```python
from build123d import *

# Parameters (mm, degrees)
EXTRUDE_THIN1_DEPTH  = 17
BOSS_EXTRUDE1_DEPTH  = 17
BOSS_EXTRUDE3_START  = 18
BOSS_EXTRUDE3_DEPTH  = 18
BOSS_EXTRUDE10_START = 18
BOSS_EXTRUDE10_DEPTH = 18
SKETCH6_W            = 4
SKETCH6_H            = 8
CUT_EXTRUDE1_DEPTH   = 1
BOSS_EXTRUDE4_DEPTH  = 18
CUT_EXTRUDE3_START   = -18
CUT_EXTRUDE3_DEPTH   = 18
BOSS_EXTRUDE5_DEPTH  = 17
BOSS_EXTRUDE6_DEPTH  = 2
SKETCH12_W           = 5
SKETCH12_H           = 1
BOSS_EXTRUDE8_DEPTH  = 33
SKETCH15_W           = 11.8
SKETCH15_H           = 8
CUT_EXTRUDE4_DEPTH   = 1
FILLET1_R            = 2
SKETCH16_W           = 30
SKETCH16_H           = 2
BOSS_EXTRUDE11_DEPTH = 18
BOSS_EXTRUDE12_START = -35
BOSS_EXTRUDE12_DEPTH = 35
SKETCH18_W           = 30
SKETCH18_H           = 35
CUT_EXTRUDE5_DEPTH   = 0.5
BOSS_EXTRUDE13_DEPTH = 2.7
BOSS_EXTRUDE14_START = -19.7
BOSS_EXTRUDE14_DEPTH = 19.7
SKETCH22_W           = 1
SKETCH22_H           = 18
BOSS_EXTRUDE15_DEPTH = 2
BOSS_EXTRUDE16_DEPTH = 19.7
BOSS_EXTRUDE17_DEPTH = 18
FILLET2_R            = 1
FILLET3_R            = 1
FILLET4_R            = 2
FILLET5_R            = 2
FILLET6_R            = 2


# Read off the part's stored shape, not the designer's step: Extrude-Thin1
with BuildPart() as part:
    # Extrude-Thin1 outline → Extrude-Thin1 (new body)
    with BuildSketch(Plane(origin=(0, 0, 0), x_dir=(1, 0, 0), z_dir=(0, 1, 0))):
        with BuildLine():
            Line((-13.736803788, -12.452377644), (-7.480049307, -32.917299422))
            Line((-7.480049307, -32.917299422), (-5.567439795, -32.332556012))
            Line((-5.567439795, -32.332556012), (-11.824194276, -11.867634235))
            ThreePointArc((-11.824194276, -11.867634235), (-11.857842102, -11.27507721), (-11.614075704, -10.733935872))
            Line((-11.614075704, -10.733935872), (-2, 1.571519877))
            Line((-2, 1.571519877), (-2, -2))
            Line((-2, -2), (32, -2))
            Line((32, -2), (32, 2.05634332))
            Line((32, 2.05634332), (34.813889941, 0.919457988))
            Line((34.813889941, 0.919457988), (35.563103127, 2.773825697))
            Line((35.563103127, 2.773825697), (30, 5.021465257))
            Line((30, 5.021465257), (30, 0))
            Line((30, 0), (0, 0))
            Line((0, 0), (0, 6.1))
            Line((0, 6.1), (-1, 6.1))
            Line((-1, 6.1), (-13.190097211, -9.502612921))
            ThreePointArc((-13.190097211, -9.502612921), (-13.824351917, -10.910606158), (-13.736803788, -12.452377644))
        make_face()
    extrude(amount=EXTRUDE_THIN1_DEPTH)

    # Sketch2 → Boss-Extrude1 (add)
    with BuildSketch(Plane(origin=(0, 17, 0), x_dir=(1, 0, 0), z_dir=(0, 1, 0))):
        Polygon((32, -2), (32, 2.05634332), (34.813889941, 0.919457988), align=None)
        Polygon((-2, -2), (-2, 1.571519877), (-5.158478254, -2.471147935), align=None)
    extrude(amount=-BOSS_EXTRUDE1_DEPTH)

    # Sketch5 → Boss-Extrude3 (add)
    with BuildSketch(Plane.XZ.offset(BOSS_EXTRUDE3_START)):
        with BuildLine():
            Line((-2, 2), (-5.158478254, 2.471147935))
            Line((-5.158478254, 2.471147935), (-11.614075704, 10.733935872))
            ThreePointArc((-11.614075704, 10.733935872), (-11.857842102, 11.27507721), (-11.824194276, 11.867634235))
            Line((-11.824194276, 11.867634235), (-5.567439795, 32.332556012))
            Line((-5.567439795, 32.332556012), (-6.523744551, 32.624927717))
            Line((-6.523744551, 32.624927717), (-12.780499032, 12.160005939))
            ThreePointArc((-12.780499032, 12.160005939), (-12.84109701, 11.092841684), (-12.402086458, 10.118274397))
            Line((-12.402086458, 10.118274397), (0, -5.755672387))
            Line((0, -5.755672387), (0, 2))
            Line((0, 2), (-2, 2))
        make_face()
    extrude(amount=-BOSS_EXTRUDE3_DEPTH)

    # Sketch14 → Boss-Extrude10 (add)
    with BuildSketch(Plane.XZ.offset(BOSS_EXTRUDE10_START)):
        with BuildLine():
            Line((0, -6.1), (-1, -6.1))
            Line((-1, -6.1), (-13.190097211, 9.502612921))
            ThreePointArc((-13.190097211, 9.502612921), (-13.824351917, 10.910606159), (-13.736803788, 12.452377644))
            Line((-13.736803788, 12.452377644), (-12.780499032, 12.160005939))
            ThreePointArc((-12.780499032, 12.160005939), (-12.84109701, 11.092841684), (-12.402086458, 10.118274397))
            Line((-12.402086458, 10.118274397), (0, -5.755672387))
            Line((0, -5.755672387), (0, -6.1))
        make_face()
    extrude(amount=-BOSS_EXTRUDE10_DEPTH)

    # Sketch6 → Cut-Extrude1 (cut)
    with BuildSketch(Plane(origin=(-15.087900976, 0, 4.612834247), x_dir=(0.2923717047227341, 0, 0.9563047559630363), z_dir=(-0.9563047559630363, 0, 0.2923717047227341))):
        with Locations((23.292015223, -9)):
            Rectangle(SKETCH6_W, SKETCH6_H)
        with Locations((13.892015223, -9)):
            Rectangle(SKETCH6_W, SKETCH6_H)
    extrude(amount=-CUT_EXTRUDE1_DEPTH, mode=Mode.SUBTRACT)

    # Sketch8 → Boss-Extrude4 (add)
    with BuildSketch(Plane.XZ):
        Polygon((30, -5.021465257), (35.563103127, -2.773825697), (34.813889941, -0.919457988), (32, 2), (30, 2), align=None)
    extrude(amount=BOSS_EXTRUDE4_DEPTH)

    # Sketch9 → Cut-Extrude3 (cut)
    with BuildSketch(Plane.XZ.offset(18).offset(CUT_EXTRUDE3_START)):
        Polygon((30, -5.021465257), (33.708735418, -3.523038884), (32.959522231, -1.668671175), (30, -2.864395772), align=None)
    extrude(amount=CUT_EXTRUDE3_DEPTH, mode=Mode.SUBTRACT)

    # Sketch10 → Boss-Extrude5 (add)
    with BuildSketch(Plane(origin=(0, 17, 0), x_dir=(1, 0, 0), z_dir=(0, 1, 0))):
        Polygon((30, 5.021465257), (25, 5.021465257), (25, 6.1), (30, 6.1), (35.937709721, 3.701009551), (35.563103127, 2.773825697), align=None)
    extrude(amount=-BOSS_EXTRUDE5_DEPTH)

    # Sketch4 → Boss-Extrude6 (add)
    with BuildSketch(Plane.XZ.offset(-17)):
        Polygon((0, 2), (0, -5.1), (5, -5.1), (5, -6.1), (0, -6.1), (-3.030429144, -6.1), (-16.354224478, 10.953680347), (-13.517385765, 13.170061658), (-11.614075704, 10.733935872), (-5.158478254, 2.471147935), (-2, 2), align=None)
    extrude(amount=BOSS_EXTRUDE6_DEPTH)

    # Sketch12 → Boss-Extrude8 (add)
    with BuildSketch(Plane.XZ.offset(-15)):
        with Locations((2.5, -5.6)):
            Rectangle(SKETCH12_W, SKETCH12_H)
    extrude(amount=BOSS_EXTRUDE8_DEPTH)

    # Sketch15 → Cut-Extrude4 (cut)
    with BuildSketch(Plane(origin=(-3.580362913, 0, -2.797286082), x_dir=(-0.6156614753256621, 0, 0.7880107536067191), z_dir=(-0.788010753606719, 0, -0.615661475325662))):
        with Locations((5.708795878, -9)):
            Rectangle(SKETCH15_W, SKETCH15_H)
    extrude(amount=-CUT_EXTRUDE4_DEPTH, mode=Mode.SUBTRACT)

    # Fillet1
    fillet1_edges = [part.edges().sort_by_distance(p)[0] for p in [
        (-1, -9, -6.1),
    ]]
    fillet(fillet1_edges, radius=FILLET1_R)

    # Sketch16 → Boss-Extrude11 (add)
    with BuildSketch(Plane.XZ):
        with Locations((15, 1)):
            Rectangle(SKETCH16_W, SKETCH16_H)
    extrude(amount=BOSS_EXTRUDE11_DEPTH)

    # Sketch17 → Boss-Extrude12 (add)
    with BuildSketch(Plane(origin=(0, 17, 0), x_dir=(1, 0, 0), z_dir=(0, 1, 0)).offset(BOSS_EXTRUDE12_START)):
        with BuildLine():
            Line((-0.672783951, -2), (-2, -2))
            Line((-2, -2), (-5.158478254, -2.471147935))
            Line((-5.158478254, -2.471147935), (-7.325420645, -5.244707716))
            ThreePointArc((-7.325420645, -5.244707716), (-4.373652198, -2.854412758), (-0.672783951, -2))
        make_face()
        with BuildLine():
            Line((-11.824194276, -11.867634235), (-10.706576434, -15.523197479))
            ThreePointArc((-10.706576434, -15.523197479), (-10.93812277, -11.445537112), (-9.260652859, -7.721691994))
            Line((-9.260652859, -7.721691994), (-11.614075704, -10.733935872))
            ThreePointArc((-11.614075704, -10.733935872), (-11.857842102, -11.27507721), (-11.824194276, -11.867634235))
        make_face()
    extrude(amount=BOSS_EXTRUDE12_DEPTH)

    # Sketch18 → Cut-Extrude5 (cut)
    with BuildSketch(Plane(origin=(0, 0, 0), x_dir=(-1, 0, 0), z_dir=(0, 0, -1))):
        with Locations((-15, -0.5)):
            Rectangle(SKETCH18_W, SKETCH18_H)
    extrude(amount=-CUT_EXTRUDE5_DEPTH, mode=Mode.SUBTRACT)

    # Sketch19 → Boss-Extrude13 (add)
    with BuildSketch(Plane(origin=(0, 17, 0), x_dir=(1, 0, 0), z_dir=(0, 1, 0))):
        with BuildLine():
            Line((5, 6.1), (25, 6.1))
            Line((25, 6.1), (30, 6.1))
            Line((30, 6.1), (35.937709721, 3.701009551))
            Line((35.937709721, 3.701009551), (34.813889941, 0.919457988))
            Line((34.813889941, 0.919457988), (32, -2))
            Line((32, -2), (-0.672783951, -2))
            ThreePointArc((-0.672783951, -2), (-4.373652198, -2.854412758), (-7.325420645, -5.244707716))
            Line((-7.325420645, -5.244707716), (-9.260652859, -7.721691994))
            ThreePointArc((-9.260652859, -7.721691994), (-10.93812277, -11.445537112), (-10.706576434, -15.523197479))
            Line((-10.706576434, -15.523197479), (-5.567439795, -32.332556012))
            Line((-5.567439795, -32.332556012), (-7.480049307, -32.917299422))
            Line((-7.480049307, -32.917299422), (-13.517385765, -13.170061658))
            Line((-13.517385765, -13.170061658), (-16.354224478, -10.953680347))
            Line((-16.354224478, -10.953680347), (-3.030429144, 6.1))
            Line((-3.030429144, 6.1), (5, 6.1))
        make_face()
    extrude(amount=BOSS_EXTRUDE13_DEPTH)

    # Sketch21 → Boss-Extrude14 (add)
    with BuildSketch(Plane(origin=(0, 19.7, 0), x_dir=(1, 0, 0), z_dir=(0, 1, 0)).offset(BOSS_EXTRUDE14_START)):
        Polygon((-4.982696385, -34.245165524), (-5.567439795, -32.332556012), (-10.062072148, -33.706703024), (-10.939187262, -30.837788757), (-12.851796774, -31.422532166), (-11.38993825, -36.204055946), align=None)
    extrude(amount=BOSS_EXTRUDE14_DEPTH)

    # Sketch22 → Boss-Extrude15 (add)
    with BuildSketch(Plane(origin=(8.564156426, 0, 28.01209347), x_dir=(0.9563047559630371, 0, -0.2923717047227314), z_dir=(0.2923717047227314, 0, 0.9563047559630371))):
        with Locations((-15.277293674, -9)):
            Rectangle(SKETCH22_W, SKETCH22_H)
    extrude(amount=BOSS_EXTRUDE15_DEPTH)

    # Sketch23 → Boss-Extrude16 (add)
    with BuildSketch(Plane(origin=(0, 19.7, 0), x_dir=(1, 0, 0), z_dir=(0, 1, 0))):
        with BuildLine():
            Line((34.813889941, 0.919457988), (35.937709721, 3.701009551))
            ThreePointArc((35.937709721, 3.701009551), (37.340267778, 3.071287576), (38.690914739, 2.336800231))
            Line((38.690914739, 2.336800231), (36.18124714, -2))
            Line((36.18124714, -2), (32, -2))
            Line((32, -2), (34.813889941, 0.919457988))
        make_face()
    extrude(amount=-BOSS_EXTRUDE16_DEPTH)

    # Sketch24 → Boss-Extrude17 (add)
    with BuildSketch(Plane.XZ):
        Polygon((36.18124714, 2), (32, 2), (34.813889941, -0.919457988), (35.563103127, -2.773825697), (38.303171931, -1.66676604), align=None)
    extrude(amount=BOSS_EXTRUDE17_DEPTH)

    # Fillet2
    fillet2_edges = [part.edges().sort_by_distance(p)[0] for p in [
        (30, -9, -2.864395772),
    ]]
    fillet(fillet2_edges, radius=FILLET2_R)

    # Fillet3
    # the kernel refuses this fillet: 1 mm, written as the material it takes off along each edge
    with BuildSketch(Plane(origin=(-13.736803788, -21.611842033, 12.452377644), x_dir=(0.956304755965878, 0, -0.29237170471343904), z_dir=(0, 1, 0))) as fillet3_piece_1:
        with BuildLine():
            CenterArc((1.222368407, 0.974962713), FILLET3_R, 154.303641792, 102.848179104)
            Line((0.321263823, 1.408564523), (0.303241732, 1.417236559))
            ThreePointArc((0.303241732, 1.417236559), (0.061834895, 0.726815775), (-0.02, 0))
            Line((-0.02, 0), (0, -0.02))
            ThreePointArc((0, -0.02), (0.5, -0.02), (0.995552632, -0.019499254))
            Line((0.995552632, -0.019499254), (1, 0))
        make_face()
    extrude(amount=21.611842033, mode=Mode.SUBTRACT)

    # Fillet4
    fillet4_edges = [part.edges().sort_by_distance(p)[0] for p in [
        (-16.354224478, 17.35, 10.953680347),
    ]]
    fillet(fillet4_edges, radius=FILLET4_R)

    # Fillet5
    fillet5_edges = [part.edges().sort_by_distance(p)[0] for p in [
        (-3.030429144, 17.35, -6.1),
    ]]
    fillet(fillet5_edges, radius=FILLET5_R)

    # Fillet6
    fillet6_edges = [part.edges().sort_by_distance(p)[0] for p in [
        (36.18124714, 0.85, 2),
    ]]
    fillet(fillet6_edges, radius=FILLET6_R)


solid = part.part
```
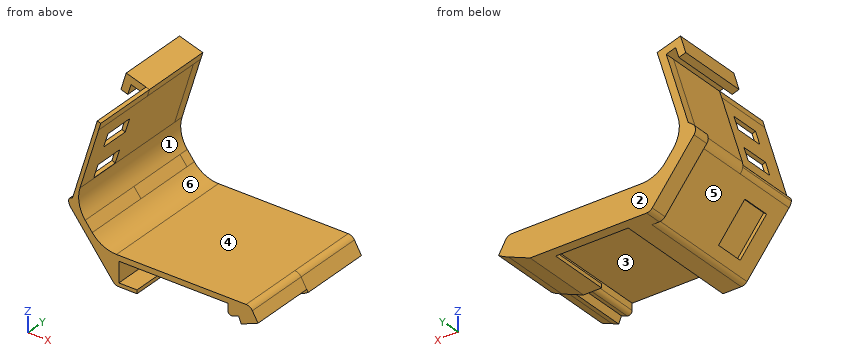
The listing builds one solid part. Answer for the finished solid, in the listing's coordinates (mm). Face numbers are marked on the shaded views. A direction names the side the tool comes from. Round coordinates to 2 decimals unless told otherwise and drop trailing zeros. Loops run counter-clockwise (first coordinate to the right, second up) from the corner with the lowest first, then second, coordinate; pieces in that order, holes last.
Q1. Find the intervals of material crossed by line 1 (Z direction, x = 4, y = 5.5); line 2 (Z direction, x = 31, y = -8.5); line 3 (Z direction, x = 24, y = 6), in increasing order.
Q2. Which of the six approach directions +Z, -Z, +X, -X, +Y, -Y give full straight-line access (tool end or side, diameter ignored) to the marked faces 4, 5 and 6?
Q3. Section C-C, the plane z = 24 is taken. Determine the outline of the cut face in (x, y).
Q4. For a pull along X with two mould halves and no side action, classify the marked faces 1, 2 and 3 as released by +X, released by -X, zero draft, split by the parting line, or undercut.
Q5. Section D-D, the plane y = -6 is taken. Count the separate pieces of the cut face and the enclosed holes in it, then the cut area to 3 significant figures.
Q6. Section B-B, the plane y = 16 is taken. Determine the outline of the cut face in (x, z) (3 decimals), then the cut area to 3 significant figures.
Q7. Section A-A, the plane x = 3.5 is taken. Determine the outline of the cut face in (y, z).
Q8. Given pin 1 Ø6 at (y, z) = (-7.5, 6) entering from -X; pin 2 Ø1.1 at (y, z) = (2.5, -5.5) entering from +X; pin 3 Ø10 at (y, z) = (-4.5, 25) entering from -X, each flat-ended and moving along its own axis, determine where each tip first touches the part or whether it passes through.
Completed:
1. line 1: z = -6.1 to -5.1, 0.5 to 2
1. line 2: z = -2.38 to 2
1. line 3: z = 0.5 to 2
2. face 4: +Z, +X, +Y, -Y
2. face 5: -Z, -X, -Y
2. face 6: +X, +Y, -Y
3. outline: (-10.21, 0) - (-9.16, 0) - (-9.16, -18) - (-8.11, -18) - (-8.11, 19.7) - (-10.21, 19.7) - close
4. face 1: released by +X
4. face 2: zero draft
4. face 3: undercut
5. separate pieces: 3
5. enclosed holes: 0
5. area: 150 mm2
6. outline: (-15.123, 9.378) - (-3.631, -5.331) arc R2 ccw to (-2.055, -6.1) - (5, -6.1) - (5, -5.1) - (0, -5.1) - (0, 0.5) - (30, 0.5) - (30, -5.021) - (25, -5.021) - (25, -6.1) - (30, -6.1) - (35.938, -3.701) arc R20.216 ccw to (38.691, -2.337) - (36.759, 1.002) arc R2 ccw to (35.028, 2) - (-0.673, 2) arc R8.442 cw to (-7.325, 5.245) - (-9.261, 7.722) arc R8.592 cw to (-10.707, 15.523) - (-4.983, 34.245) - (-11.39, 36.204) - (-12.852, 31.423) - (-10.939, 30.838) - (-10.062, 33.707) - (-7.48, 32.917) - (-13.517, 13.17) - (-14.778, 12.185) arc R2 ccw to start
6. area: 267 mm2
7. outline: (-18, -6.1) - (19.7, -6.1) - (19.7, 2) - (-18, 2) - (-18, 0.5) - (17, 0.5) - (17, -5.1) - (-18, -5.1) - close
8. pin 1: stops at x = -12.8
8. pin 2: stops at x = 32.85
8. pin 3: stops at x = -10.57
